```python
from build123d import *

# Parameters (mm, degrees)
SKETCH_1_W          = 62
SKETCH_1_H          = 62
SKETCH_1_R          = 12.5
EXTRUDE_1_DEPTH     = 5
CHAMFER_1_SIZE      = 3
SKETCH_2_R          = 1.6
CUT_EXTRUDE_1_DEPTH = 45.124822946


with BuildPart() as part:
    # ｽｹｯﾁ1 → ﾎﾞｽ - 押し出し1 (new body)
    with BuildSketch(Plane.XY):
        Rectangle(SKETCH_1_W, SKETCH_1_H)
        Circle(SKETCH_1_R, mode=Mode.SUBTRACT)
    extrude(amount=EXTRUDE_1_DEPTH)

    # 面取り1
    chamfer_1_edges = [part.edges().sort_by_distance(p)[0] for p in [
        (-31, 31, 2.5),
        (31, 31, 2.5),
        (31, -31, 2.5),
        (-31, -31, 2.5),
    ]]
    chamfer(chamfer_1_edges, length=CHAMFER_1_SIZE)

    # ｽｹｯﾁ2 → ｶｯﾄ - 押し出し1 (cut, through all)
    with BuildSketch(Plane.XY.offset(5)):
        with Locations((27, 27)):
            Circle(SKETCH_2_R)
        with Locations(Location((-27, 27, 0), (0, 0, 180))):
            Circle(SKETCH_2_R)
        with Locations(Location((27, -27, 0), (0, 0, 180))):
            Circle(SKETCH_2_R)
        with Locations((-27, -27)):
            Circle(SKETCH_2_R)
    extrude(amount=-CUT_EXTRUDE_1_DEPTH, mode=Mode.SUBTRACT)


solid = part.part
```
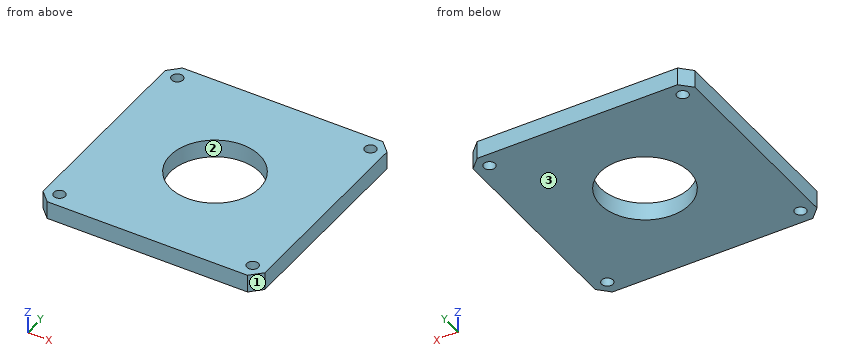
Input: part model. Units: mm. Frame: model coordinates. Face numbers are marked on the shaded views. Give positions to 0.01 mm unless a question says otherwise; leave off trailing zeros. Order: outer loops, then holes, each group sorted by start corner. A loop starts at its lowest first (then second) coordinate and runs counter-clockwise, first axis right, second up.
1. Cut plane A-A (x = 27). Return loops of the section in (y, z).
Computed:
outline: (-31, 0) - (-28.6, 0) - (-28.6, 5) - (-31, 5) - close; (-25.4, 0) - (25.4, 0) - (25.4, 5) - (-25.4, 5) - close; (28.6, 0) - (31, 0) - (31, 5) - (28.6, 5) - close
2. Cut plane B-B (y = 0). Return loops of the section in (x, z).
Computed:
outline: (-31, 0) - (-12.5, 0) - (-12.5, 5) - (-31, 5) - close; (12.5, 0) - (31, 0) - (31, 5) - (12.5, 5) - close
3. Pin query (flat end, axial travel): pin 1 Ø3.5 at (x, y) = (-27, -27) entering from -Z; pin 2 Ø3 at (x, y) = (27, -27) entering from -Z. Return the tip coordinate at first contact, or that it passes through.
Computed:
pin 1: stops at z = 0
pin 2: passes through
4. Cut plane C-C (z = 3.2). Return loops of the section in (x, y), and give its area (3 significant figures).
Computed:
outline: (-31, -28) - (-28, -31) - (28, -31) - (31, -28) - (31, 28) - (28, 31) - (-28, 31) - (-31, 28) - close; hole circle Ø3.2 at (-27, -27); hole circle Ø3.2 at (-27, 27); hole circle Ø25 at (0, 0); hole circle Ø3.2 at (27, -27); hole circle Ø3.2 at (27, 27)
area: 3,300 mm2
5. Line query: probe 1 along Y at (x, z) = (27, 3.4); probe 2 along Y at (x, z) = (0, 2.3); probe 3 along Y at (x, z) = (-26.5, 4.7). Output: solid intervals per line, ascending.
Computed:
probe 1: y = -31 to -28.6, -25.4 to 25.4, 28.6 to 31
probe 2: y = -31 to -12.5, 12.5 to 31
probe 3: y = -31 to -28.52, -25.48 to 25.48, 28.52 to 31
6. Draft query along X for the marked faces 1, 2 and 3. Return one class per face: released by +X, released by -X, zero draft, split by the parting line, or undercut.
Computed:
face 1: released by +X
face 2: undercut
face 3: zero draft
